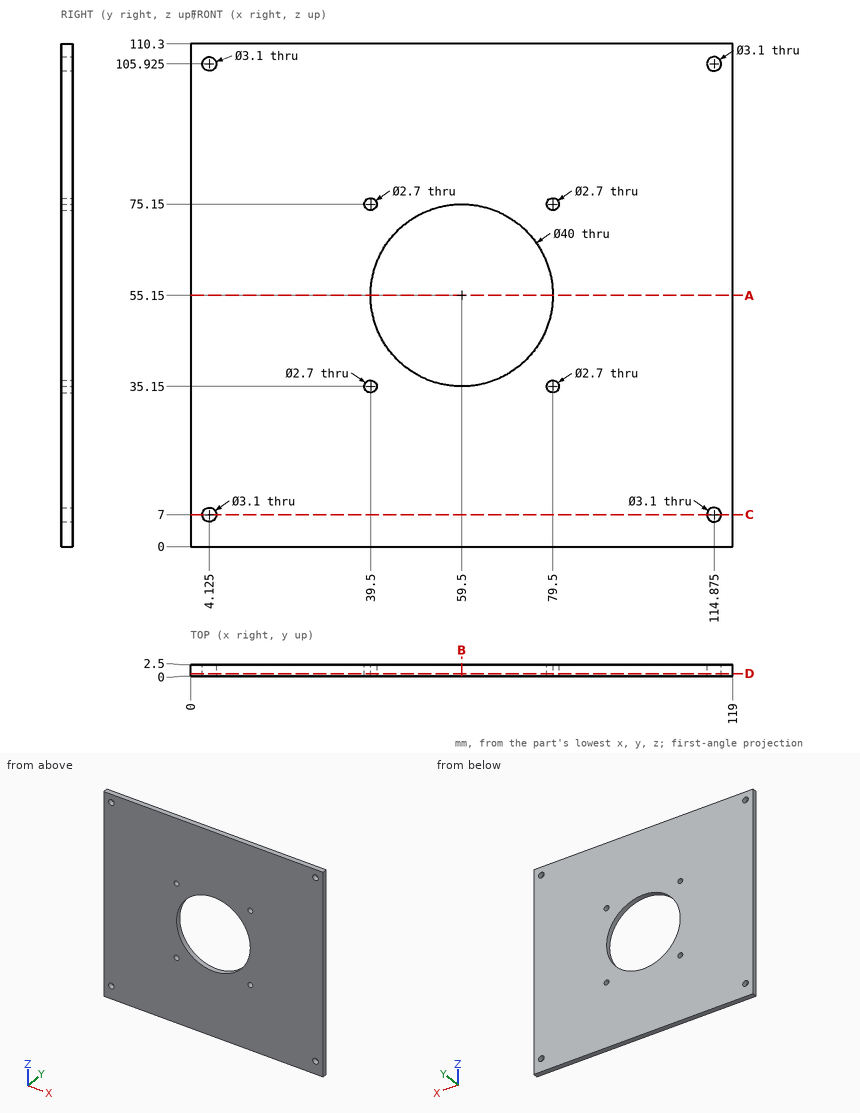
Design review of the part shown in the three views and the two pictorial views. Dimensions are in mm from the part's minimum x, y and z. Coordinates: 2 decimals unless noted, no trailing zeros. Loops run counter-clockwise (first coordinate to the right, second up) from the corner with the lowest first, then second, coordinate; pieces in that order, holes last. Notation, with made-up numbers: M 36,-5.75 L 64,-5.75 A22 ccw 64,20.25 Z; hole C -21.75,-30 d9. An arc over 180 degrees is marked long. Put each result on its own line as item: value. Start each with the question number.
Q1. Add section C-C (z = 7). Write out the cut boundary in (x, y) (3 decimals), and give its area (3 significant figures).
Q2. Add section A-A (z = 55.15). Write out the cut boundary in (x, y).
Q3. Wall thickness on line 1 (X direction, y = 1, z = 7) (3 decimals); line 2 (X direction, y = 0.9, z = 35); line 3 (X direction, y = 0.35, z = 56): over which ranges is each line inside the solid? List them lowest first.
Q4. Add section B-B (x = 59.5). Write out the cut boundary in (y, z), and give its area (3 significant figures).
Q5. Clearance check with a flat-ended pin moving along its axis: pin 1 (3 mm diameter, centred on x = 114.875, z = 105.925, fed in from -Y). State where the tip first meets the part, or that it passes through.
Q6. Add section D-D (y = 0.5). Count the separate pieces of the cut face and the enclosed holes in it, and give its area (3 significant figures).
Answers:
1. outline: M 0,0 L 2.575,0 L 2.575,2.5 L 0,2.5 Z; M 5.675,0 L 113.325,0 L 113.325,2.5 L 5.675,2.5 Z; M 116.425,0 L 119,0 L 119,2.5 L 116.425,2.5 Z
1. area: 282 mm^2
2. outline: M 0,0 L 39.5,0 L 39.5,2.5 L 0,2.5 Z; M 79.5,0 L 119,0 L 119,2.5 L 79.5,2.5 Z
3. line 1: x = 0 to 2.575, 5.675 to 113.325, 116.425 to 119
3. line 2: x = 0 to 38.16, 40.84 to 78.16, 80.84 to 119
3. line 3: x = 0 to 39.52, 79.48 to 119
4. outline: M 0,0 L 2.5,0 L 2.5,35.15 L 0,35.15 Z; M 0,75.15 L 2.5,75.15 L 2.5,110.3 L 0,110.3 Z
4. area: 176 mm^2
5. pin 1: passes through
6. separate pieces: 1
6. enclosed holes: 9
6. area: 11,800 mm^2
